Verification items for the finished model (mm, model axes). A direction names the side the tool comes from. Round coordinates to 2 decimals unless told otherwise and drop trailing zeros. Loops run counter-clockwise (first coordinate to the right, second up) from the corner with the lowest first, then second, coordinate; pieces in that order, holes last.
Autodesk Inventor part; units mm, degrees
ref_plane "YZ Plane" through (0, 0, 0) normal (1, 0, 0) x (0, 1, 0)
ref_plane "XZ Plane" through (0, 0, 0) normal (0, 1, 0) x (-1, 0, 0)
ref_plane "XY Plane" through (0, 0, 0) normal (0, 0, 1) x (1, 0, 0)
sketch "Эскиз1" plane through (0, 0, 0) normal (0, 1, 0) x (-1, 0, 0)
  line L0 (-6.0731, 25) -> (3.9269, 25)
  line L1 (-6.0731, -62) -> (-6.0731, 25)
  line L2 (3.9269, 31.5) -> (7.9269, 31.5)
  line L3 (7.9269, 31.5) -> (7.9269, -68.5)
  line L4 (3.9269, 25) -> (3.9269, 31.5)
  line L5 (-6.0731, 25) -> (-2.5731, 25)
  line L6 (-2.5731, 25) -> (-2.5731, 27.5)
  line L7 (-2.5731, 27.5) -> (-6.0731, 27.5)
  line L8 (-6.0731, 27.5) -> (-6.0731, 25)
  line L9 (3.9269, 27.5) -> (5.9269, 27.5)
  line L10 (5.9269, 27.5) -> (5.9269, 31.5)
  line L11 (5.9269, 31.5) -> (3.9269, 31.5)
  line L12 (3.9269, 31.5) -> (3.9269, 27.5)
  line L13 (7.9269, -18.5) -> (10, -18.5)
  line L14 (-6.0731, -62) -> (3.9269, -62)
  line L15 (3.9269, -68.5) -> (7.9269, -68.5)
  line L16 (3.9269, -62) -> (3.9269, -68.5)
  line L17 (-6.0731, -62) -> (-2.5731, -62)
  line L18 (-2.5731, -62) -> (-2.5731, -64.5)
  line L19 (-2.5731, -64.5) -> (-6.0731, -64.5)
  line L20 (-6.0731, -64.5) -> (-6.0731, -62)
  line L21 (3.9269, -64.5) -> (5.9269, -64.5)
  line L22 (5.9269, -64.5) -> (5.9269, -68.5)
  line L23 (5.9269, -68.5) -> (3.9269, -68.5)
  line L24 (3.9269, -68.5) -> (3.9269, -64.5)
  point P0 (0, 0)
  point P1 (-2.5731, 25)
  dimension "d0" = 14
  dimension "d1" = 6.5
  dimension "d2" = 6.5
  dimension "d3" = 2.5
  dimension "d4" = 4
  dimension "d5" = 2
  dimension "d6" = 100
  dimension "d7" = 50
extrude "Выдавливание1" add sketch "Эскиз1" along normal blind 712 contours L8 L7 L6 L0 | L0 L4 L9 L10 L2 L3 L15 L22 L21 L16 L14 L1 | L14 L18 L19 L20
sketch "Эскиз5" plane through (-5.9269, 0, 31.5) normal (0, 0, 1) x (1, 0, 0)
  line L0 (-2, 0) -> (12, 0)
  line L1 (12, 0) -> (12, 16)
  line L2 (12, 16) -> (-2, 16)
  line L3 (-2, 16) -> (-2, 0)
  line L4 (-2, 0) -> (-2, 712)
  line L5 (12, 712) -> (8.5, 712)
  line L6 (12, 712) -> (-2, 712)
  line L7 (-2, 712) -> (-2, 696)
  line L8 (-2, 696) -> (12, 696)
  line L9 (12, 696) -> (12, 712)
  point P0 (5.9269, 0)
  dimension "d18" = 16
  dimension "d19" = 0
  dimension "d20" = 16
extrude "Выдавливание3" add sketch "Эскиз5" against normal blind 100
sketch "Эскиз6" plane through (-7.9269, 0, 31.5) normal (0, 0, 1) x (1, 0, 0)
  line L0 (14, 25.5) -> (4, 25.5)
  line L1 (14, 25.5) -> (10.5, 25.5)
  line L2 (10.5, 25.5) -> (10.5, 28)
  line L3 (10.5, 28) -> (14, 28)
  line L4 (14, 28) -> (14, 25.5)
  line L5 (4, 32) -> (0, 32)
  line L6 (2, 28) -> (2, 32)
  line L7 (2, 32) -> (4, 32)
  line L8 (4, 32) -> (4, 28)
  line L9 (4, 25.5) -> (4, 32)
  line L10 (4, 28) -> (2, 28)
  line L11 (14, 38.5) -> (4, 38.5)
  line L12 (14, 38.5) -> (10.5, 38.5)
  line L13 (10.5, 36) -> (14, 36)
  line L14 (14, 36) -> (14, 38.5)
  line L15 (10.5, 38.5) -> (10.5, 36)
  line L16 (4, 36) -> (2, 36)
  line L17 (2, 36) -> (2, 32)
  line L18 (4, 32) -> (4, 36)
  line L19 (4, 38.5) -> (4, 32)
  line L20 (14, 36) -> (14, 28)
  line L21 (14, 16) -> (14, 696)
  line L22 (14, 356) -> (16, 356)
  line L23 (0, 0) -> (14, 0)
  line L24 (14, 686.5) -> (4, 686.5)
  line L25 (14, 686.5) -> (10.5, 686.5)
  line L26 (10.5, 684) -> (14, 684)
  line L27 (14, 684) -> (14, 686.5)
  line L28 (10.5, 686.5) -> (10.5, 684)
  line L29 (4, 684) -> (2, 684)
  line L30 (4, 680) -> (0, 680)
  line L31 (2, 684) -> (2, 680)
  line L32 (2, 680) -> (4, 680)
  line L33 (4, 680) -> (4, 684)
  line L34 (4, 686.5) -> (4, 680)
  line L35 (14, 673.5) -> (4, 673.5)
  line L36 (14, 673.5) -> (10.5, 673.5)
  line L37 (10.5, 676) -> (14, 676)
  line L38 (14, 676) -> (14, 673.5)
  line L39 (10.5, 673.5) -> (10.5, 676)
  line L40 (4, 676) -> (2, 676)
  line L41 (2, 676) -> (2, 680)
  line L42 (4, 680) -> (4, 676)
  line L43 (4, 673.5) -> (4, 680)
  line L44 (14, 676) -> (14, 684)
  point P0 (7.9269, 0)
  dimension "d26" = 356
extrude "Выдавливание4" cut sketch "Эскиз6" against normal blind 100 contours L0 L9 L8 L18 L19 L11 L15 L13 L20 L3 L2 | L37 L39 L35 L43 L42 L33 L34 L24 L28 L26 L21
chamfer "Фаска2" distance 4.99 angle 45 8 edges at (4.3231, 684, 27.5) (4.3231, 676, 27.5) (4.3231, 36, 27.5) (4.3231, 28, 27.5) (4.3231, 36, -64.5) (4.3231, 28, -64.5) (4.3231, 684, -64.5) (4.3231, 676, -64.5)
sketch "Эскиз7" plane through (6.0731, 40.99, 27.5) normal (1, 0, 0) x (0, 0, -1)
  circle A0 centre (76, 51.01) radius 2.5
  circle A1 centre (16, 51.01) radius 2.5
  line L0 (-4, -24.99) -> (-4, 655.01)
  line L1 (96, -24.99) -> (96, 655.01)
  line L2 (-4, -40.99) -> (96, -40.99)
  circle A2 centre (76, -36.99) radius 2.5
  circle A3 centre (16, -36.99) radius 2.5
  point P0 (27.5, -40.99)
  dimension "d32" = 5
  dimension "d33" = 20
  dimension "d34" = 20
  dimension "d35" = 5
  dimension "d36" = 92
  dimension "d37" = 92
  dimension "d38" = 5
  dimension "d39" = 5
  dimension "d40" = 4
  dimension "d41" = 4
ref_plane "РабПлоскость1" through (0, 356, 0) normal (0, -1, 0) x (1, 0, 0)
hole "Отверстие1" at (6.0731, 4, 11.5) at (6.0731, 4, -48.5) at (6.0731, 92, -48.5) at (6.0731, 92, 11.5) direction (-1, 0, 0) diameter 5 end through all counterbore diameter 9 counterbore depth 7
mirror "Зеркальное отражение1" about plane through (0, 356, 0) normal (0, -1, 0) of "Отверстие1"
fillet "Сопряжение2" radius 2 8 edges at (2.5731, 0, -50.5616) (2.5731, 0, -46.4384) (2.5731, 0, 9.4384) (2.5731, 0, 13.5616) (2.5731, 712, -50.5616) (2.5731, 712, -46.4384) (2.5731, 712, 9.4384) (2.5731, 712, 13.5616)
sketch "Sketch8" plane through (6.0731, 40.99, 27.5) normal (1, 0, 0) x (0, 0, -1)
  line L0 (96, -40.99) -> (-4, -40.99)
  circle A0 centre (46, -40.99) radius 17
  line L1 (96, 671.01) -> (-4, 671.01)
  line L2 (29, -40.99) -> (63, -40.99)
  line L3 (63, -40.99) -> (63, 671.01)
  line L4 (63, 671.01) -> (29, 671.01)
  line L5 (29, 671.01) -> (29, -40.99)
  point P0 (27.5, -40.99)
  dimension "d51" = 34
extrude "Extrusion5" add sketch "Sketch8" against normal blind 10 contours A0 L5 L1 L3
properties part number "TopPaz" material "Алюминий 6061"
1. Scan lines: L1, parallel to Z at x = 3, y = 4; L2, parallel to Y at x = 2.25, z = -49.5; L3, parallel to Z at x = -4.75, y = 92. Record each from-to range of solid material in increasing order.
2. Tool access check on faces 4 (the face through (2.573, 26, -51)), 5 (the face through (-7, 354, -68.5)), 6 (the face through (2.573, 686, 14)). Record the directions out of +Z, -Z, +X, -X, +Y, -Y that give a thin tool (end or side, any length) a straight path to the whole face; none if there is none.
3. Section check A-A (y = 541). Enter the section's corners in (x, z), then the cut area to 3 significant figures.
4. Gauge pin test, flat ends, axial feed: P1, Ø2, axis at x = 0, y = 20.5, coming from the +Z side; P2, Ø1.8, axis at x = 5, z = -53.5, coming from the +Y side; P3, Ø1, axis at x = 3, z = -44.5, coming from the -Y side; P4, Ø4, axis at y = 92, z = -48.5, coming from the +X side. Record the tip position at first contact, or that the pin passes through.
5. Release check for a two-part mould opening along X. For faces 1 (the face through (2.573, 26, 14)), 2 (the face through (6.073, 351, -18)), 3 (the face through (-1, 0, -18)) record: released by +X, released by -X, zero draft, split by the parting line, or undercut.
Taken from the geometry:
1. L1: z = -68.5 to -53, -44 to 7, 16 to 31.5
1. L2: y = 8.39 to 25.5, 38.5 to 87.61, 96.39 to 615.61, 624.39 to 673.5, 686.5 to 703.61
1. L3: z = -64.5 to -51, -46 to 9, 14 to 27.5
2. face 4: -Z
2. face 5: -Z, +X, -X, +Y, -Y
2. face 6: +Z
3. outline: (-7.93, -68.5) - (-5.93, -68.5) - (-5.93, -64.5) - (-3.93, -64.5) - (-3.93, -62) - (2.57, -62) - (2.57, -64.5) - (6.07, -64.5) - (6.07, 27.5) - (2.57, 27.5) - (2.57, 25) - (-3.93, 25) - (-3.93, 27.5) - (-5.93, 27.5) - (-5.93, 31.5) - (-7.93, 31.5) - close
3. area: 1,270 mm2
4. P1: stops at z = 25
4. P2: stops at y = 711.98
4. P3: stops at y = 0.92
4. P4: passes through
5. face 1: undercut
5. face 2: released by +X
5. face 3: zero draft
